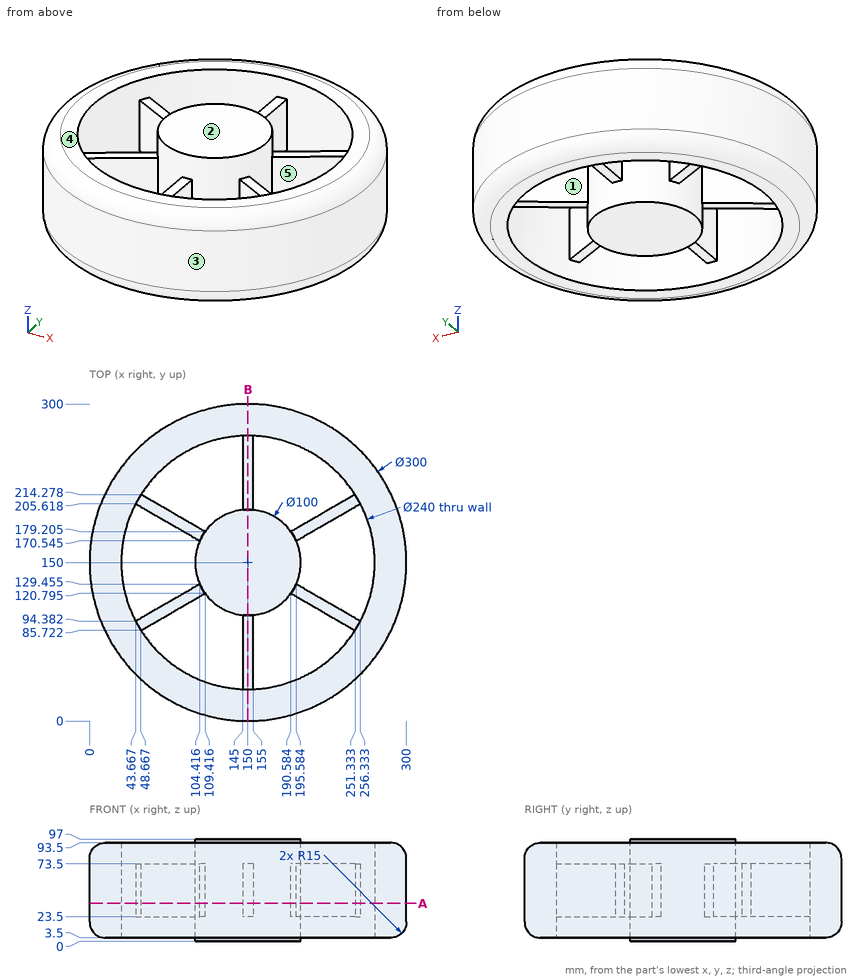
For this review, use the dimensioned drawing (mm, ordinates from the lowest corner) and the shaded views. A direction names the side the tool comes from. Give positions to 0.01 mm unless a question says otherwise; leave off trailing zeros. Order: outer loops, then holes, each group sorted by start corner. A loop starts at its lowest first (then second) coordinate and runs counter-clockwise, first axis right, second up. Notation, with made-up numbers: M -26,59.25 L -5,59.25 A17 ccw -5,63.25 Z; hole C 45,61.25 d3. An arc over 180 degrees is marked long. One line per question, with ' | ' between items. Start each with the question number.
1) Consider section B-B, the plane x = 150. Give the boundary of the cut face in (y, z).
2) Mouldability with a two-part tool opening along X and no side actions: class the marked faces 3, 4 and 5 as pulls with the +X half, pulls with the -X half, needs draft (parallel to the pull), parting line crosses it, or undercut.
3) For the marked faces 1 and 2, list the 3-axis set-ups (+Z, -Z, +X, -X, +Y, -Y) from which the entire face can be reached by the end or side of a thin tool; tool diameter is ignored.
4) Clearance check with flat-ended pins moving along their axes: P1, Ø8, axis at x = 151.5, y = 219, coming from the -Z side; P2, Ø1.5, axis at y = 81, z = 80, coming from the -X side; P3, Ø5, axis at x = 187.5, z = 53, coming from the -Y side; P4, Ø1.5, axis at x = 265.5, y = 126, coming from the +Z side (3 decimals). State where each tip first meets the part, or that it passes through.
5) Wall thickness on L1, parallel to Y at x = 152, z = 19.5; L2, parallel to Y at x = 181, z = 12.5 (1 decimal); L3, parallel to X at y = 116.5, z = 89.5: over which ranges is each line inside the solid? List them lowest first. Write a range as from..to.
6) Consider section A-A, the plane z = 36. State how many separate pieces and enclosed holes the cut face has, then the cut area to 3 significant figures.
Found:
1) outline: M 0,18.5 A15 ccw 15,3.5 L 30,3.5 L 30,23.5 L 100,23.5 L 100,0 L 200,0 L 200,23.5 L 270,23.5 L 270,3.5 L 285,3.5 A15 ccw 300,18.5 L 300,78.5 A15 ccw 285,93.5 L 270,93.5 L 270,73.5 L 200,73.5 L 200,97 L 100,97 L 100,73.5 L 30,73.5 L 30,93.5 L 15,93.5 A15 ccw 0,78.5 Z
2) face 3: parting line crosses it | face 4: needs draft | face 5: undercut
3) face 1: +Z, -Z | face 2: +Z, +X, -X, +Y, -Y
4) P1: stops at z = 23.5 | P2: stops at x = 16.5 | P3: stops at y = 4.14 | P4: passes through
5) L1: y = 0.01..30.02, 100.04..199.96, 269.98..299.99 | L2: y = 4.5..34.1, 110.8..189.2, 265.9..295.5 | L3: x = 8.72..34.77, 112.88..187.12, 265.23..291.28
6) separate pieces: 1 | enclosed holes: 6 | area: 37,500 mm²
